Check sheet for the modelled part. Datum: model origin and axes. Units: mm. A direction names the side the tool comes from. Give positions to 0.01 mm unless a question says otherwise; leave off trailing zeros. Write each loop counter-clockwise with the first axis right and the second up, starting at its lowest first coordinate (ties: lowest second). Pieces come first, ordered by that corner, then holes.
from build123d import *

# Parameters (mm, degrees)
SKETCH_1_W          = 75
SKETCH_1_H          = 45
EXTRUDE_1_DEPTH     = 19
SKETCH_2_W          = 10
SKETCH_2_H          = 45
CUT_EXTRUDE_1_DEPTH = 14
SKETCH_3_W          = 47
SKETCH_3_H          = 45
CUT_EXTRUDE_2_DEPTH = 16
SKETCH_4_R          = 1.5
SKETCH_4_R_2        = 7.5
CUT_EXTRUDE_3_DEPTH = 48.681233206
SKETCH_5_W          = 14
SKETCH_5_H          = 38
CUT_EXTRUDE_4_DEPTH = 48.681233206
FILLET_1_R          = 30
CHAMFER_1_SIZE      = 1.5
SKETCH_8_W          = 36
SKETCH_8_H          = 24
CUT_EXTRUDE_6_DEPTH = 48.681233206
FILLET_2_R          = 3
SKETCH_9_R          = 1.5
CUT_EXTRUDE_7_DEPTH = 46.918405896
FILLET_3_R          = 3
FILLET_4_R          = 4


with BuildPart() as part:
    # 草图1 → 凸台-拉伸1 (new body)
    with BuildSketch(Plane(origin=(0, 0, 0), x_dir=(1, 0, 0), z_dir=(0, 1, 0))):
        Rectangle(SKETCH_1_W, SKETCH_1_H)
    extrude(amount=EXTRUDE_1_DEPTH)

    # 草图2 → 切除-拉伸1 (cut)
    with BuildSketch(Plane.XZ):
        with Locations((-32.5, 0)):
            Rectangle(SKETCH_2_W, SKETCH_2_H)
        with Locations((32.5, 0)):
            Rectangle(SKETCH_2_W, SKETCH_2_H)
    extrude(amount=-CUT_EXTRUDE_1_DEPTH, mode=Mode.SUBTRACT)

    # 草图3 → 切除-拉伸2 (cut)
    with BuildSketch(Plane(origin=(0, 19, 0), x_dir=(1, 0, 0), z_dir=(0, 1, 0))):
        Rectangle(SKETCH_3_W, SKETCH_3_H)
    extrude(amount=-CUT_EXTRUDE_2_DEPTH, mode=Mode.SUBTRACT)

    # 草图4 → 切除-拉伸3 (cut, through all)
    with BuildSketch(Plane.XZ):
        with Locations(Location((10.606601718, 10.606601718, 0), (0, 0, 270))):
            Circle(SKETCH_4_R)
        with Locations(Location((10.606601718, -10.606601718, 0), (0, 0, 270))):
            Circle(SKETCH_4_R)
        with Locations(Location((-10.606601718, -10.606601718, 0), (0, 0, 270))):
            Circle(SKETCH_4_R)
        with Locations(Location((-10.606601718, 10.606601718, 0), (0, 0, 270))):
            Circle(SKETCH_4_R)
        with Locations(Location((0, 0, 0), (0, 0, 270))):
            Circle(SKETCH_4_R_2)
    extrude(amount=-CUT_EXTRUDE_3_DEPTH, mode=Mode.SUBTRACT)

    # 草图5 → 切除-拉伸4 (cut, through all)
    with BuildSketch(Plane(origin=(0, 19, 0), x_dir=(1, 0, 0), z_dir=(0, 1, 0))):
        with Locations((30.5, -3.5)):
            Rectangle(SKETCH_5_W, SKETCH_5_H)
    extrude(amount=-CUT_EXTRUDE_4_DEPTH, mode=Mode.SUBTRACT)

    # 圆角1
    fillet_1_edges = [part.edges().sort_by_distance(p)[0] for p in [
        (23.5, 1.5, 22.5),
    ]]
    fillet(fillet_1_edges, radius=FILLET_1_R)

    # 倒角1
    chamfer_1_edges = [part.edges().sort_by_distance(p)[0] for p in [
        (-10.606601718, 3, 12.106601718),
        (-10.606601718, 3, -9.106601718),
        (10.606601718, 3, -9.106601718),
        (10.606601718, 3, 12.106601718),
    ]]
    chamfer(chamfer_1_edges, length=CHAMFER_1_SIZE)

    # 草图8 → 切除-拉伸6 (cut, through all)
    with BuildSketch(Plane.XZ):
        with Locations((-37.5, 0)):
            Rectangle(SKETCH_8_W, SKETCH_8_H)
    extrude(amount=-CUT_EXTRUDE_6_DEPTH, mode=Mode.SUBTRACT)

    # 圆角2
    fillet_2_edges = [part.edges().sort_by_distance(p)[0] for p in [
        (-19.5, 1.5, 12),
        (-19.5, 1.5, -12),
    ]]
    fillet(fillet_2_edges, radius=FILLET_2_R)

    # 草图9 → 切除-拉伸7 (cut, through all)
    with BuildSketch(Plane.XZ.offset(-14)):
        with Locations(Location((32.5, -19, 0), (0, 0, 270))):
            Circle(SKETCH_9_R)
        with Locations(Location((-32.5, -19, 0), (0, 0, 270))):
            Circle(SKETCH_9_R)
        with Locations(Location((-32.5, 19, 0), (0, 0, 270))):
            Circle(SKETCH_9_R)
    extrude(amount=-CUT_EXTRUDE_7_DEPTH, mode=Mode.SUBTRACT)

    # 圆角3
    fillet_3_edges = [part.edges().sort_by_distance(p)[0] for p in [
        (-37.5, 16.5, 12),
        (-37.5, 16.5, -12),
        (-37.5, 16.5, 22.5),
        (-37.5, 16.5, -22.5),
        (37.5, 16.5, -22.5),
        (37.5, 16.5, -15.5),
    ]]
    fillet(fillet_3_edges, radius=FILLET_3_R)

    # 圆角4
    fillet_4_edges = [part.edges().sort_by_distance(p)[0] for p in [
        (23.5, 1.5, -15.5),
    ]]
    fillet(fillet_4_edges, radius=FILLET_4_R - 0.0001)  # a hair under: the kernel refuses the full size


solid = part.part
1) Access from +Z, -Z, +X, -X, +Y, -Y to the whole of each face (thin tool, end or side, straight path). Record for faces 1 (the flat face through (23.5, 11, -19)), 2 (the cylindrical face through (-33.4, 16.5, -17.8)), 3 (the cylindrical face through (-20.36, 1.52, -11.1)).
2) Sectioned sample at B-B on y = 4. Record the boundary of the cut face in (x, z).
3) Scan lines: L1, parallel to Z at x = 11, y = 2.75; L2, parallel to X at y = 15.5, z = 20; L3, parallel to Y at x = 15, z = -0.5. Record each from-to range of solid material in increasing order.
4) Draft check along X on faces 4 (the flat face through (-33, 14, 17)), 5 (the cylindrical face through (0.33, 1.479, 7.493)), 6 (the cylindrical face through (-36.6, 16.46, -12.86)). Enter one of: +X half, -X half, draft (parallel to the pull), parting line (faces both ways), or undercut.
5) Sectioned sample at C-C on z = 0. Record the boundary of the cut face in (x, y).
6) Gauge pin test, flat ends, axial feed: pin 1 (5.5 mm diameter, centred on x = 30.5, y = 14, fed in from +Z); pin 2 (13.5 mm diameter, centred on x = 0, z = 0, fed in from -Y); pin 3 (2 mm diameter, centred on y = 3.5, z = 11.5, fed in from -X); pin 4 (3 mm diameter, centred on y = 15, z = 14.5, fed in from -X). Record the tip position at first contact, or that the pin passes through.
7) Sectioned sample at A-A on x = -24.5. Record the boundary of the cut face in (y, z), then the cut area to 3 significant figures.
8) Sectioned sample at D-D on x = -32.5. Record the boundary of the cut face in (y, z).
Answers below:
1. face 1: +Z, -Z, +Y
1. face 2: +Y, -Y
1. face 3: -X, +Y, -Y
2. outline: (-27.5, -22.5) - (-23.5, -22.5) - (-23.5, -12) - (-27.5, -12) - close; (-27.5, 12) - (-23.5, 12) - (-23.5, 22.5) - (-27.5, 22.5) - close; (23.5, -22.5) - (27.5, -22.5) - (27.5, -15.5) - (23.5, -15.5) - close
3. L1: z = -22.5 to -13.33, -7.88 to 7.88, 13.33 to 16.87
3. L2: x = -37.46 to -33.62, -31.38 to -23.5
3. L3: y = 0 to 3
4. face 4: draft
4. face 5: undercut
4. face 6: -X half
5. outline: (-19.5, 0) - (-7.5, 0) - (-7.5, 3) - (-19.5, 3) - close; (7.5, 0) - (22.55, 0) - (22.55, 3) - (7.5, 3) - close
6. pin 1: stops at z = -15.5
6. pin 2: passes through
6. pin 3: stops at x = -27.5
6. pin 4: stops at x = -37.5
7. outline: (0, -22.5) - (19, -22.5) - (19, -12) - (0, -12) - close; (0, 12) - (19, 12) - (19, 22.5) - (0, 22.5) - close
7. area: 399 mm2
8. outline: (14, -22.5) - (19, -22.5) - (19, -20.5) - (14, -20.5) - close; (14, -17.5) - (19, -17.5) - (19, -12) - (14, -12) - close; (14, 12) - (19, 12) - (19, 17.5) - (14, 17.5) - close; (14, 20.5) - (19, 20.5) - (19, 22.5) - (14, 22.5) - close
